Autodesk Inventor part; units mm, degrees
ref_plane "YZ Plane" through (0, 0, 0) normal (1, 0, 0) x (0, 1, 0)
ref_plane "XZ Plane" through (0, 0, 0) normal (0, 1, 0) x (-1, 0, 0)
ref_plane "XY Plane" through (0, 0, 0) normal (0, 0, 1) x (1, 0, 0)
sketch "Boceto1" plane through (0, 0, 0) normal (0, 1, 0) x (-1, 0, 0)
  arc A0 (-18, 72.808) -> (20, 72.2842) centre (0, 0) ccw
  line L0 (-18, 72.808) -> (-18, 72.2842)
  line L1 (-11, 25) -> (13, 25)
  line L2 (55, 8) -> (40, 8)
  line L3 (40, 8) -> (40, -42)
  line L4 (40, -42) -> (55, -42)
  line L5 (55, -42) -> (55, 8)
  line L6 (-40, 8) -> (-55, 8)
  line L7 (-55, 8) -> (-55, -42)
  line L8 (-55, -42) -> (-40, -42)
  line L9 (-40, -42) -> (-40, 8)
  line L10 (20, 72.2842) -> (13, 72.2842)
  line L11 (13, 72.2842) -> (13, 25)
  line L12 (-18, 72.808) -> (-11, 72.808)
  line L13 (-11, 72.808) -> (-11, 25)
  line L14 (-18, 72.2842) -> (-18, 72.808)
  dimension "d0" = 150
  dimension "d2" = 18
  dimension "d3" = 25
  dimension "d4" = 15
  dimension "d5" = 50
  dimension "d6" = 15
  dimension "d7" = 50
  dimension "d8" = 40
  dimension "d9" = 40
  dimension "d63" = 8
  dimension "d64" = 8
extrude "Extrusión1" add sketch "Boceto1" along normal blind 2
sketch "Boceto2" plane through (0, 0, 0) normal (0, 1, 0) x (-1, 0, 0)
  arc A0 (-18, 72.808) -> (20, 72.2842) centre (0, 0) ccw
  line L0 (-18, 72.808) -> (-18, 72.2842)
  line L1 (20, 72.2842) -> (13, 72.2842)
  line L2 (-18, 72.808) -> (-11, 72.808)
  line L3 (-11, 72.808) -> (-11, 72.2842)
  line L4 (-18, 72.2842) -> (-18, 72.808)
  line L5 (20, 72.2842) -> (13, 72.2842)
  line L6 (13, 72.2842) -> (20, 72.2842)
  line L7 (64.5832, 27.0002) -> (13, 27.0002)
  line L8 (13, 27.0002) -> (13, 72.2842)
  line L9 (-11, 72.2842) -> (-20, 72.2842)
  line L10 (-64.5832, 27.0002) -> (-11, 27.0002)
  line L11 (-11, 27.0002) -> (-11, 72.2842)
  arc A1 (69.8214, 4.9968) -> (69.8214, -4.9968) centre (70, 0) ccw
  arc A2 (-69.8214, -4.9968) -> (-69.8214, 4.9968) centre (-70, 0) ccw
  arc A3 (4.9968, -69.8214) -> (-4.9968, -69.8214) centre (0, -70) ccw
  arc A4 (4.9968, -69.8214) -> (69.8214, -4.9968) centre (0, 0) ccw
  arc A5 (69.8214, 4.9968) -> (64.5832, 27.0002) centre (0, 0) ccw
  arc A6 (-64.5832, 27.0002) -> (-69.8214, 4.9968) centre (0, 0) ccw
  arc A7 (-69.8214, -4.9968) -> (-4.9968, -69.8214) centre (0, 0) ccw
  dimension "d14" = 150
  dimension "d45" = 10
  dimension "d46" = 10
  dimension "d47" = 10
extrude "Extrusión2" add sketch "Boceto2" against normal blind 32 contours L9 L11 L10 A6 A2 A7 A3 A4 A1 A5 L7 L8 L1 A0
sketch "Boceto3" plane through (0, 0, 0) normal (0, 1, 0) x (-1, 0, 0)
  line L0 (-40, 8) -> (-40, -42)
  line L1 (-40, -3) -> (-15, -3)
  line L2 (-15, -3) -> (-15, -31)
  line L3 (-15, -31) -> (-40, -31)
  line L4 (-40, -31) -> (-40, -3)
  line L5 (39.9026, -3) -> (14.9026, -3)
  line L6 (14.9026, -3) -> (14.9026, -31)
  line L7 (14.9026, -31) -> (39.9026, -31)
  line L8 (39.9026, -31) -> (39.9026, -3)
  line L9 (-40, 8) -> (-55, 8)
  line L10 (55, 8) -> (40, 8)
  point P0 (0, 0)
  dimension "d27" = 25
  dimension "d28" = 28
  dimension "d30" = 25
  dimension "d31" = 28
  dimension "d65" = 11
  dimension "d66" = 11
extrude "Extrusión3" add sketch "Boceto3" against normal blind 11
sketch "Boceto4" plane through (0, 0, 0) normal (0, 1, 0) x (-1, 0, 0)
  line L0 (34, 26.7953) -> (43.9649, 26.7953)
  line L1 (43.9649, 26.7953) -> (43.9649, 8)
  line L2 (40, -2.9415) -> (34, -2.9415)
  line L3 (34, -2.9415) -> (34, 26.7953)
  line L4 (13, 27.0002) -> (13, 72.2842)
  line L5 (55, 8) -> (40, 8)
  line L6 (40, 8) -> (40, -42)
  line L7 (43.9649, 8) -> (40, 8)
  line L8 (40, 8) -> (40, -2.9415)
  line L9 (43.9649, 5.0585) -> (44, 5.0585)
  point P0 (0, 0)
  dimension "d37" = 21
extrude "Extrusión4" add sketch "Boceto4" against normal blind 32
sketch "Boceto5" plane through (0, 0, 0) normal (1, 0, 0) x (0, 1, 0)
  circle A0 centre (-16, 51.2842) radius 11
  line L0 (0, 72.2842) -> (-32, 72.2842)
  line L1 (2, -75) -> (2, 72.808)
  point P0 (0, 0)
  point P1 (2, 72.2842)
  dimension "d40" = 22
  dimension "d41" = 21
  dimension "d42" = 18
extrude "Extrusión5" cut sketch "Boceto5" along normal mid plane 38
sketch "Boceto6" plane through (0, 0, 0) normal (0, 1, 0) x (-1, 0, 0)
  arc A0 (69.8214, 4.9968) -> (69.8214, -4.9968) centre (70, 0) ccw
  circle A1 centre (70, 0) radius 1.5
  circle A2 centre (0, -70) radius 1.5
  circle A3 centre (-70, 0) radius 1.5
  line L0 (64.5832, 27.0002) -> (13, 27.0002)
  line L1 (-11, 27.0002) -> (-64.5832, 27.0002)
  point P0 (0, 0)
  dimension "d48" = 3
  dimension "d49" = 3
  dimension "d50" = 3
extrude "Extrusión6" cut sketch "Boceto6" against normal blind 33
sketch "Boceto8" plane through (0, 0, 0) normal (0, 1, 0) x (-1, 0, 0)
  line L0 (59.5508, 67.2842) -> (-59.748, 67.2842)
  line L1 (-59.748, 67.2842) -> (-59.748, 82.2842)
  line L2 (-59.748, 82.2842) -> (59.5508, 82.2842)
  line L3 (59.5508, 82.2842) -> (59.5508, 67.2842)
  line L4 (13, 72.2842) -> (20, 72.2842)
  point P0 (0, 0)
  dimension "d67" = 15
  dimension "d71" = 5
extrude "Extrusión8" cut sketch "Boceto8" along normal mid plane 70
sketch "Boceto9" plane through (0, 0, 0) normal (0, 1, 0) x (-1, 0, 0)
  line L0 (-64.5832, 27.0002) -> (-11, 27.0002)
  line L1 (-23, 27.0002) -> (-64.5832, 27.0002)
  line L2 (-40.2309, 57.2842) -> (-23, 57.2842)
  line L3 (-23, 57.2842) -> (-23, 27.0002)
  line L4 (-11, 67.2842) -> (-11, 27.0002)
  line L5 (-33.1337, 67.2842) -> (-11, 67.2842)
  line L6 (25, 27.0002) -> (64.5832, 27.0002)
  line L7 (40.2309, 57.2842) -> (25, 57.2842)
  line L8 (25, 57.2842) -> (25, 27.0002)
  line L9 (13, 27.0002) -> (13, 67.2842)
  line L10 (13, 67.2842) -> (33.1337, 67.2842)
  arc A0 (-40.2309, 57.2842) -> (-64.5832, 27.0002) centre (0, 0) ccw
  arc A1 (64.5832, 27.0002) -> (40.2309, 57.2842) centre (0, 0) ccw
  dimension "d73" = 12
  dimension "d76" = 10
  dimension "d77" = 12
  dimension "d78" = 10
extrude "Extrusión9" cut sketch "Boceto9" against normal blind 32
sketch "Boceto10" plane through (0, 0, 0) normal (0, 1, 0) x (-1, 0, 0)
  line L0 (-23, 57.2842) -> (-40.2309, 57.2842)
  circle A0 centre (-40.2309, 57.2842) radius 4
  arc A1 (69.8214, 4.9968) -> (40.2309, 57.2842) centre (0, 0) ccw
  circle A2 centre (40.2309, 57.2842) radius 4
  line L1 (25, 57.2842) -> (25, 27.0002)
  circle A3 centre (25, 57.2842) radius 4
  line L2 (-23, 27.0002) -> (-23, 57.2842)
  circle A4 centre (-23, 57.2842) radius 4
  line L3 (-11, 67.2842) -> (-11, 27.0002)
  dimension "d81" = 8
  dimension "d82" = 8
  dimension "d83" = 8
  dimension "d84" = 8
extrude "Extrusión10" add sketch "Boceto10" against normal blind 32
sketch "Boceto11" plane through (0, 0, 0) normal (0, 1, 0) x (-1, 0, 0)
  line L0 (-27, 57.2842) -> (-36.2309, 57.2842)
  arc A0 (-43.4373, 54.8927) -> (-36.2309, 57.2842) centre (-40.2309, 57.2842) ccw
  arc A1 (-27, 57.2842) -> (-23, 53.2842) centre (-23, 57.2842) ccw
  circle A2 centre (-23, 57.2842) radius 1.5
  arc A3 (25, 53.2842) -> (29, 57.2842) centre (25, 57.2842) ccw
  circle A4 centre (25, 57.2842) radius 1.5
  arc A5 (36.2309, 57.2842) -> (43.4373, 54.8927) centre (40.2309, 57.2842) ccw
  circle A6 centre (40.2309, 57.2842) radius 1.5
  circle A7 centre (-40.2309, 57.2842) radius 1.5
  point P0 (0, 0)
  dimension "d89" = 3
  dimension "d90" = 3
  dimension "d91" = 3
  dimension "d92" = 3
extrude "Extrusión11" cut sketch "Boceto11" against normal blind 32
sketch "Boceto12" plane through (0, 0, 0) normal (1, 0, 0) x (0, 1, 0)
  circle A0 centre (-16, 12.0585) radius 4
  line L0 (0, 54.8927) -> (0, 4.9968)
  line L1 (0, -2.9415) -> (-32, -2.9415)
  circle A1 centre (-5, 12.0585) radius 1.5
  line L2 (-32, 67.2842) -> (-32, -75)
  circle A2 centre (-27, 12.0585) radius 1.5
  circle A3 centre (-16, 2.0585) radius 1.5
  circle A4 centre (-16, 20.5585) radius 1.5
  point P0 (0, 0)
  dimension "d95" = 8
  dimension "d96" = 16
  dimension "d97" = 15
  dimension "d98" = 3
  dimension "d99" = 5
  dimension "d102" = 3
  dimension "d103" = 5
  dimension "d104" = 3
  dimension "d105" = 5
  dimension "d106" = 3
  dimension "d107" = 16
  dimension "d108" = 16
  dimension "d109" = 15
  dimension "d110" = 23.5
extrude "Extrusión12" cut sketch "Boceto12" against normal blind 50
sketch "Boceto13" plane through (0, 0, 0) normal (0, 1, 0) x (-1, 0, 0)
  line L0 (-11, 67.2842) -> (-11, 27.0002)
  line L1 (-19, 62.2842) -> (-19, 40.2842)
  line L2 (-11, 62.2842) -> (-19, 62.2842)
  line L3 (-19, 62.2842) -> (-19, 40.2842)
  line L4 (-19, 40.2842) -> (-11, 40.2842)
  line L5 (-11, 40.2842) -> (-11, 62.2842)
  point P0 (0, 0)
extrude "Extrusión13" cut sketch "Boceto13" along normal mid plane 32
sketch "Boceto14" plane through (0, 0, 0) normal (1, 0, 0) x (0, 1, 0)
  circle A0 centre (-2, 55.2842) radius 1.5
  line L0 (2, -75) -> (2, 67.2842)
  line L1 (2, 67.2842) -> (-32, 67.2842)
  circle A1 centre (-2, 47.2842) radius 1.5
  point P0 (0, 0)
  dimension "d118" = 3
  dimension "d119" = 4
  dimension "d120" = 12
  dimension "d121" = 3
  dimension "d122" = 4
  dimension "d123" = 20
extrude "Extrusión14" cut sketch "Boceto14" along normal blind 29
properties part number "Cuerpo" material "Nilón 6/6"
For this review, take the finished solid that the model builds, in its own axes (mm). A direction names the side the tool comes from. Give positions to 0.01 mm unless a question says otherwise; leave off trailing zeros. Loops run counter-clockwise (first coordinate to the right, second up) from the corner with the lowest first, then second, coordinate; pieces in that order, holes last.
Item 1: Take a section at C-C, the plane z = -48. State the section outline as (x, y) points, and give its area (3 significant figures).
Item 2: Tool access review of faces 5 (the cylindrical face through (-68.134, -15.776, 16.057)), 6 (the flat face through (-19, -16, 51)): name each direction out of +Z, -Z, +X, -X, +Y, -Y from which nothing blocks a thin tool from reaching the whole face with its end or side.
Item 3: Insertion check: pin 1 (5 mm diameter, centred on x = -25, z = -2, fed in from -Y); pin 2 (6 mm diameter, centred on x = 38.5, z = 2, fed in from -Y); pin 3 (1 mm diameter, centred on x = 46, y = 0.5, fed in from +Z). Each pin has a flat end and moves straight along its axis. Give the tip position at first contact, or say it passes through.
Item 4: Draft analysis for pull direction X (two halves, no side actions). For faces 1 (the cylindrical face through (-38.91, -18.95, 14.76)), 2 (the flat face through (32, -16, 57.284)), 3 (the flat face through (1, 2, -3)), 4 (the cylindrical face through (-2.818, -15.238, -74.947)), state which applies: +X half, -X half, draft (parallel to the pull), parting line (faces both ways), or undercut.
Item 5: Take a section at B-B, the plane z = -25. State the section outline as (x, y) points.
Item 6: Take a section at A-A, the plane x = -47.5. State the section outline as (y, z) points.
Item 7: For line 1 along X through (y, z) = (-21.5, 20); line 2 along Z through (x, y) = (0, -13.5); line 3 along Z through (x, y) = (-14, -16), list the stretches that pass through material, from the lowest coordinate up.
Calculated:
1. outline: (-57.63, -32) - (-50.95, -32) - (-50.95, 0) - (50.95, 0) - (50.95, -32) - (57.63, -32) - (57.63, 2) - (-57.63, 2) - close
1. area: 658 mm2
2. face 5: -Y
2. face 6: none
3. pin 1: stops at y = -11
3. pin 2: stops at y = 0
3. pin 3: stops at z = 59.62
4. face 1: undercut
4. face 2: undercut
4. face 3: draft
4. face 4: parting line
5. outline: (-70.71, -32) - (-65.38, -32) - (-65.38, 0) - (-55, 0) - (-55, 2) - (-70.71, 2) - close; (-40, 0) - (-39.9, 0) - (-39.9, -11) - (-14.9, -11) - (-14.9, 0) - (15, 0) - (15, -11) - (40, -11) - (40, 2) - (-40, 2) - close; (55, 0) - (65.38, 0) - (65.38, -32) - (70.71, -32) - (70.71, 2) - (55, 2) - close
6. outline: (-32, -58.04) - (2, -58.04) - (2, -42) - (0, -42) - (0, -51.42) - (-32, -51.42) - close; (-32, 51.42) - (0, 51.42) - (0, 8) - (2, 8) - (2, 58.04) - (-32, 58.04) - close
7. line 1: x = -72.28 to -67.08, -43.96 to -34, 67.08 to 72.28
7. line 2: z = -75 to -71.5, -68.5 to -65
7. line 3: z = -73.68 to -68.59, 27 to 40.28, 62.28 to 67.28
